Input: part model. Units: mm. Frame: model coordinates. Coordinates: 2 decimals unless noted, no trailing zeros. Order: outer loops, then holes, each group sorted by start corner. A loop starts at its lowest first (then second) coordinate and runs counter-clockwise, first axis right, second up. Notation, with made-up numbers: (5.25, -14.5) - (36.25, -14.5) arc R24 ccw to (36.25, 15.5) - close; hole circle Ø4 at (8, -2.75). An arc over 180 degrees is marked (long way). Answer as CSV lines item,"result". Start each with the question number.
Item 1: Material intervals for line 1 along X through (y, z) = (0.3, -10); line 2 along X through (y, z) = (0.6, -10.5); line 3 along Z through (x, y) = (-15.5, 0.65), sorted ascending.
Item 2: Section B-B (z = -10). Output: boundary loops of the cut face in (x, y).
Item 3: Section A-A (y = 0.3). Output: boundary loops of the cut face in (x, z).
Item 4: Draft query along X for faces 1 (the cylindrical face through (-15.1, 0.5, -46)), 2 (the cylindrical face through (-12.5, 0.5, 19.9)), 3 (the flat face through (-25.328, 0.493, -31.015)). Return one class per face: +X half, -X half, draft (parallel to the pull), parting line (faces both ways), or undercut.
Item 5: Section C-C (x = -15). Output: boundary loops of the cut face in (y, z).
Item 6: Section D-D (z = 20). Output: boundary loops of the cut face in (x, y).
Autodesk Inventor part; units mm, degrees
ref_plane "YZ Plane" through (0, 0, 0) normal (1, 0, 0) x (0, 1, 0)
ref_plane "XZ Plane" through (0, 0, 0) normal (0, 1, 0) x (-1, 0, 0)
ref_plane "XY Plane" through (0, 0, 0) normal (0, 0, 1) x (1, 0, 0)
sketch "Sketch1" plane through (0, 0, 0) normal (0, 1, 0) x (-1, 0, 0)
  line L0 (0, 0) -> (30, 0)
  line L1 (30, 0) -> (30, -20)
  line L2 (30, -20) -> (0, -20)
  line L3 (0, -20) -> (0, 0)
  line L4 (30, -10) -> (0, -10)
  line L5 (15, 0) -> (15, -20)
  circle A0 centre (25, -10) radius 2
  circle A1 centre (15, -40) radius 2.5
  circle A2 centre (5, -10) radius 2
  line L6 (30, 0) -> (0, 0)
  arc A3 (9.4763, -42.3428) -> (20.5237, -42.3428) centre (15, -40) ccw
  line L7 (30, -20) -> (20.5237, -42.3428)
  line L8 (0, -20) -> (9.4763, -42.3428)
  line L9 (30, 0) -> (0, 0)
  circle A4 centre (15, 20) radius 2.5
  arc A5 (20.5237, 22.3428) -> (9.4763, 22.3428) centre (15, 20) ccw
  line L10 (30, 0) -> (20.5237, 22.3428)
  line L11 (0, 0) -> (9.4763, 22.3428)
  dimension "d0" = 20
  dimension "d1" = 30
  dimension "d2" = 5
  dimension "d3" = 4
  dimension "d5" = 20
  dimension "d6" = 5
  dimension "d11" = 12
extrude "Extrusion2" add sketch "Sketch1" along normal blind 1 contours L11 A5 L10 L0 | L0 L5 L4 A2 L3 | L0 L1 L4 A0 L5 | L4 A2 L5 L2 L3 | L4 A0 L1 L2 L5 | L2 L7 A3 L8
properties part number "Platte2"
Determined:
1,line 1,"x = -30 to -27, -23 to -7, -3 to 0"
1,line 2,"x = -30 to -26.94, -23.06 to -6.94, -3.06 to 0"
1,line 3,"z = -45.98 to -42.45, -37.55 to 17.55, 22.45 to 25.98"
2,outline,"(-30, 0) - (-27, 0) - (-27, 1) - (-30, 1) - close; (-23, 0) - (-7, 0) - (-7, 1) - (-23, 1) - close; (-3, 0) - (0, 0) - (0, 1) - (-3, 1) - close"
3,outline,"(-30, -20) - (-20.52, -42.34) arc R6 ccw to (-9.48, -42.34) - (0, -20) - (0, 0) - (-9.48, 22.34) arc R6 ccw to (-20.52, 22.34) - (-30, 0) - close; hole circle Ø4 at (-25, -10); hole circle Ø5 at (-15, -40); hole circle Ø5 at (-15, 20); hole circle Ø4 at (-5, -10)"
4,face 1,"parting line"
4,face 2,"undercut"
4,face 3,"-X half"
5,outline,"(0, -46) - (1, -46) - (1, -42.5) - (0, -42.5) - close; (0, -37.5) - (1, -37.5) - (1, 17.5) - (0, 17.5) - close; (0, 22.5) - (1, 22.5) - (1, 26) - (0, 26) - close"
6,outline,"(-21.52, 0) - (-17.5, 0) - (-17.5, 1) - (-21.52, 1) - close; (-12.5, 0) - (-8.48, 0) - (-8.48, 1) - (-12.5, 1) - close"
